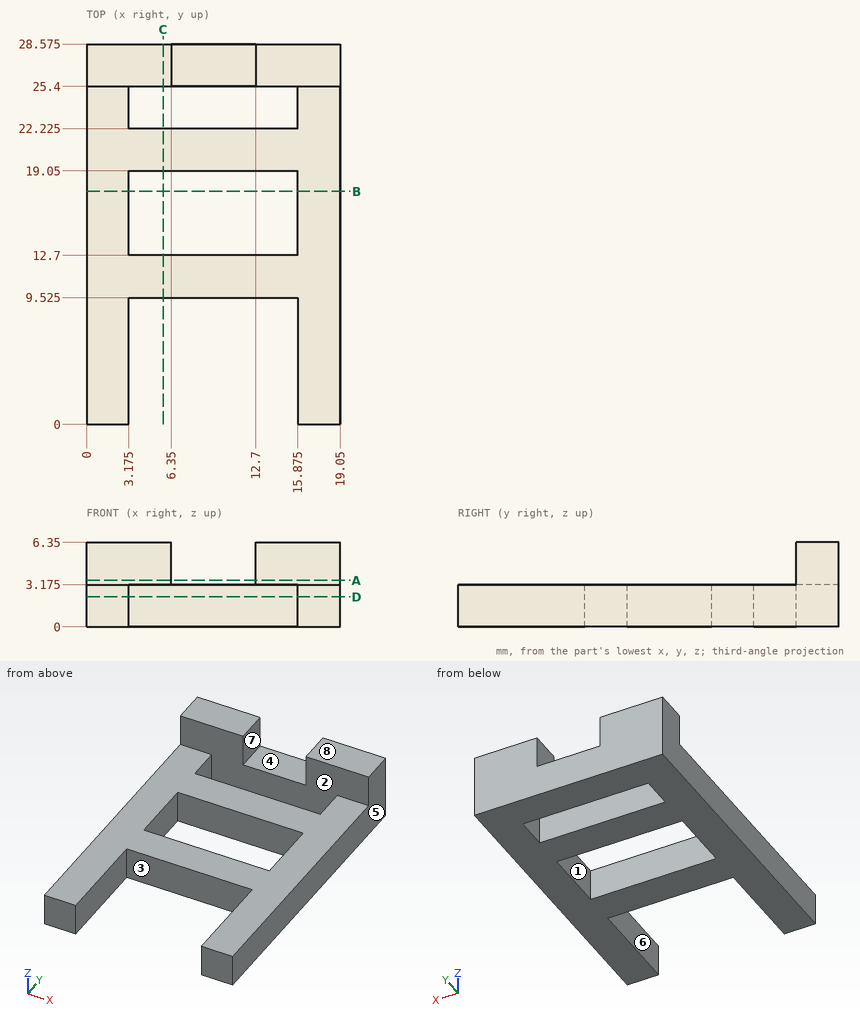
The drawing under review shows one solid part. Ordinate dimensions are in mm from its lowest x, y, z. A direction names the side the tool comes from. Coordinates: 2 decimals unless noted, no trailing zeros. Loops run counter-clockwise (first coordinate to the right, second up) from the corner with the lowest first, then second, coordinate; pieces in that order, holes last.
Item 1: Add section D-D (z = 2.25). Write out the cut boundary in (x, y) (3 decimals), and give its area (3 significant figures).
Completed:
outline: (0, 0) - (3.175, 0) - (3.175, 9.525) - (15.875, 9.525) - (15.875, 0) - (19.05, 0) - (19.05, 28.575) - (0, 28.575) - close; hole (3.175, 12.7) - (15.875, 12.7) - (15.875, 19.05) - (3.175, 19.05) - close; hole (3.175, 22.225) - (15.875, 22.225) - (15.875, 25.4) - (3.175, 25.4) - close
area: 302 mm2
Item 2: For the marked faces 1, 2, 3 and 4, list the 3-axis set-ups (+Z, -Z, +X, -X, +Y, -Y) from which the entire face can be reached by the end or side of a thin tool; tool diameter is ignored.
Completed:
face 1: +Z, -Z
face 2: +Z
face 3: +Z, -Z, -Y
face 4: +Z, +Y, -Y
Item 3: Wall thickness on L1, parallel to Y at x = 8.5, z = 0.5 (3 decimals); L2, parallel to X at y = 18, z = 0.5 (3 decimals); L3, parallel to Z at x = 1.75, y = 6.25 (3 decimals): over which ranges is each line inside the solid? List them lowest first.
Completed:
L1: y = 9.525 to 12.7, 19.05 to 22.225, 25.4 to 28.575
L2: x = 0 to 3.175, 15.875 to 19.05
L3: z = 0 to 3.175
Item 4: Add section B-B (y = 17.5). Write out the cut boundary in (x, z) (3 decimals), and give its area (3 significant figures).
Completed:
outline: (0, 0) - (3.175, 0) - (3.175, 3.175) - (0, 3.175) - close; (15.875, 0) - (19.05, 0) - (19.05, 3.175) - (15.875, 3.175) - close
area: 20.2 mm2
Item 5: Draft analysis for pull direction X (two halves, no side actions). For the marked faces 5, 6, 7 and 8, state which applies: pulls with the +X half, pulls with the -X half, needs draft (parallel to the pull), parting line crosses it, or undercut.
Completed:
face 5: pulls with the +X half
face 6: undercut
face 7: undercut
face 8: needs draft
Item 6: Add section A-A (z = 3.5). Write out the cut boundary in (x, y) (3 decimals).
Completed:
outline: (0, 25.4) - (6.35, 25.4) - (6.35, 28.575) - (0, 28.575) - close; (12.7, 25.4) - (19.05, 25.4) - (19.05, 28.575) - (12.7, 28.575) - close
Item 7: Clearance check with flat-ended pins moving along their axes: pin 1 (2 mm diameter, centred on x = 8, z = 4, fed in from -Y) (3 decimals); pin 2 (1.6 mm diameter, centred on x = 10.5, y = 27.5, fed in from +Z) (3 decimals). State where each tip first meets the part, or that it passes through.
Completed:
pin 1: stops at y = 9.525
pin 2: stops at z = 3.175
Item 8: Add section C-C (x = 5.75). Write out the cut boundary in (y, z) (3 decimals).
Completed:
outline: (9.525, 0) - (12.7, 0) - (12.7, 3.175) - (9.525, 3.175) - close; (19.05, 0) - (22.225, 0) - (22.225, 3.175) - (19.05, 3.175) - close; (25.4, 0) - (28.575, 0) - (28.575, 6.35) - (25.4, 6.35) - close
